```python
from build123d import *

# Parameters (mm, degrees)
F0_W     = 58
F0_H     = 32.5
F0_R     = 5
F0_H_2   = 15
F1_DEPTH = 15
F2_R     = 7.5
F3_DEPTH = 30


with BuildPart() as f1:
    # F0 (on Top) → F1 (new body)
    with BuildSketch(Plane.XY):
        with Locations((0, 23.75)):
            Rectangle(F0_W, F0_H)
        with Locations((-21, 27)):
            Circle(F0_R, mode=Mode.SUBTRACT)
        with Locations((21, 27)):
            Circle(F0_R, mode=Mode.SUBTRACT)
        Rectangle(F0_W, F0_H_2)
        with Locations((0, -23.75)):
            Rectangle(F0_W, F0_H)
        with Locations((-21, -27)):
            Circle(F0_R, mode=Mode.SUBTRACT)
        with Locations((21, -27)):
            Circle(F0_R, mode=Mode.SUBTRACT)
    extrude(amount=F1_DEPTH)

    # F2 (on Right) → F3 (cut, symmetric)
    with BuildSketch(Plane.YZ):
        Circle(F2_R)
    extrude(amount=F3_DEPTH, both=True, mode=Mode.SUBTRACT)


solid = f1.part
```
Can you work these out from the model? Positions are in its coordinate system, mm. Coordinates: 2 decimals unless noted, no trailing zeros. Loops run counter-clockwise (first coordinate to the right, second up) from the corner with the lowest first, then second, coordinate; pieces in that order, holes last.
1) I need wall thicknesses on probe 1 along Y at (x, z) = (21, 9.5); probe 2 along X at (y, z) = (25, 11.75); probe 3 along Y at (x, z) = (21, 4). Which ranges of each line are inside material? Lowest first, please.
2) Imagine slicing it at D-D on z = 11.5. List the corners of the cut face in (x, y) for me.
3) For pin 1 (6 mm diameter, centred on x = -21, y = 27, fed in from -Z), with a flat end and sliding along its axis, tell me the tip position at first contact or that it passes through.
4) Imagine slicing it at C-C on y = 27. List the corners of the cut face in (x, z) for me.
5) Imagine slicing it at A-A on x = 21. List the corners of the cut face in (y, z) for me.
6) Thinking about a two-plate mould opening in X: for faces 1 (the flat face through (0, -24, 0)), 2 (the flat face through (29, -1, 9)), 3 (the flat face through (-29, 1, 9)), 4 (the cylindrical face through (-22.08, -31.88, 7.4)), which applies, pulls with the +X half, pulls with the -X half, needs draft (parallel to the pull), parting line crosses it, or undercut?
7) Imagine slicing it at B-B on z = 1.5. List the corners of the cut face in (x, y) for me, plus the area to 3 significant figures.
Completed:
1. probe 1: y = -40 to -32, -22 to 22, 32 to 40
1. probe 2: x = -29 to -25.58, -16.42 to 16.42, 25.58 to 29
1. probe 3: y = -40 to -32, -22 to -6.34, 6.34 to 22, 32 to 40
2. outline: (-29, -40) - (29, -40) - (29, 40) - (-29, 40) - close; hole circle Ø10 at (-21, -27); hole circle Ø10 at (-21, 27); hole circle Ø10 at (21, -27); hole circle Ø10 at (21, 27)
3. pin 1: passes through
4. outline: (-29, 0) - (-26, 0) - (-26, 15) - (-29, 15) - close; (-16, 0) - (16, 0) - (16, 15) - (-16, 15) - close; (26, 0) - (29, 0) - (29, 15) - (26, 15) - close
5. outline: (-40, 0) - (-32, 0) - (-32, 15) - (-40, 15) - close; (-22, 0) - (-7.5, 0) arc R7.5 cw to (7.5, 0) - (22, 0) - (22, 15) - (-22, 15) - close; (32, 0) - (40, 0) - (40, 15) - (32, 15) - close
6. face 1: needs draft
6. face 2: pulls with the +X half
6. face 3: pulls with the -X half
6. face 4: undercut
7. outline: (-29, -40) - (29, -40) - (29, -7.35) - (-29, -7.35) - close; (-29, 7.35) - (29, 7.35) - (29, 40) - (-29, 40) - close; hole circle Ø10 at (-21, -27); hole circle Ø10 at (-21, 27); hole circle Ø10 at (21, -27); hole circle Ø10 at (21, 27)
7. area: 3,470 mm2
